Job drawing, mm, ordinate dimensions from the low corner. One solid piece. Give positions to 0.01 mm unless a question says otherwise; leave off trailing zeros. Order: outer loops, then holes, each group sorted by start corner. A loop starts at its lowest first (then second) coordinate and runs counter-clockwise, first axis right, second up. Notation, with made-up numbers: M 39,-8.5 L 70,-8.5 A18 cw 70,26.5 Z; hole C 26,73.25 d6. An arc over 180 degrees is marked long. One line per question, with ' | ' between items.
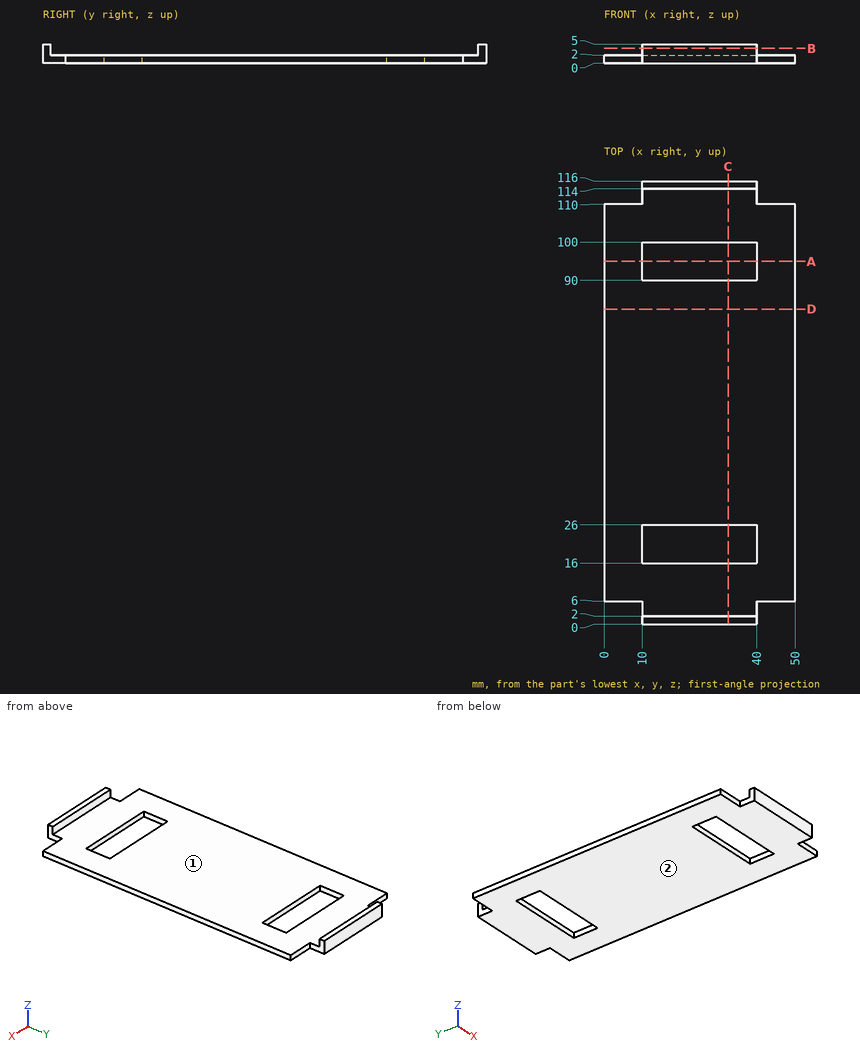
1. Drop flat-ended pins along their axis: pin 1 (3 mm diameter, centred on x = 15, y = 50.5, fed in from +Z); pin 2 (1.5 mm diameter, centred on y = 2.5, z = 2.5, fed in from -X); pin 3 (1 mm diameter, centred on x = 7, z = 1, fed in from -Y). Give the stop position or say it passes through.
Worked out:
pin 1: stops at z = 2 | pin 2: stops at x = 10 | pin 3: stops at y = 6
2. Probe L1, parallel to Y at x = 21, z = 1.4; L2, parallel to Y at x = 32, z = 3.4; L3, parallel to Z at x = 45.5, y = 106.5. List the from-to ranges inside material, lowest first. Write a range as from..to.
Worked out:
L1: y = 0..16, 26..90, 100..116 | L2: y = 0..2, 114..116 | L3: z = 0..2
3. Slice it at C-C on x = 32.5. Give the cut face in (y, z), then the cut area to 3 significant figures.
Worked out:
outline: M 0,0 L 16,0 L 16,2 L 2,2 L 2,5 L 0,5 Z; M 26,0 L 90,0 L 90,2 L 26,2 Z; M 100,0 L 116,0 L 116,5 L 114,5 L 114,2 L 100,2 Z | area: 204 mm2
4. Slice it at A-A on y = 95. Give the cut face in (x, z), then the cut area to 3 significant figures.
Worked out:
outline: M 0,0 L 10,0 L 10,2 L 0,2 Z; M 40,0 L 50,0 L 50,2 L 40,2 Z | area: 40.0 mm2
5. Slice it at D-D on y = 82.5. Give the cut face in (x, z), then the cut area to 3 significant figures.
Worked out:
outline: M 0,0 L 50,0 L 50,2 L 0,2 Z | area: 100 mm2
6. Slice it at B-B on z = 3.85. Give the cut face in (x, y), then the cut area to 3 significant figures.
Worked out:
outline: M 10,0 L 40,0 L 40,2 L 10,2 Z; M 10,114 L 40,114 L 40,116 L 10,116 Z | area: 120 mm2
7. Mould opens along Y. For the marked faces 1 and 2 say: released by +Y, released by -Y, zero draft, split by the parting line, or undercut.
Worked out:
face 1: undercut | face 2: zero draft
